Design review of the part shown in the three views and the two pictorial views. Dimensions are in mm from the part's minimum x, y and z. A direction names the side the tool comes from. Coordinates: 2 decimals unless noted, no trailing zeros. Write each loop counter-clockwise with the first axis right and the second up, starting at its lowest first coordinate (ties: lowest second). Pieces come first, ordered by that corner, then holes. Notation, with made-up numbers: (72, -33.5) -> (128, -33.5) arc R35 cw to (128, -0.5) -> close; hole circle Ø2 at (-34, 19). An arc over 180 degrees is marked (long way). Write item = value, one per line. Start each with the question number.
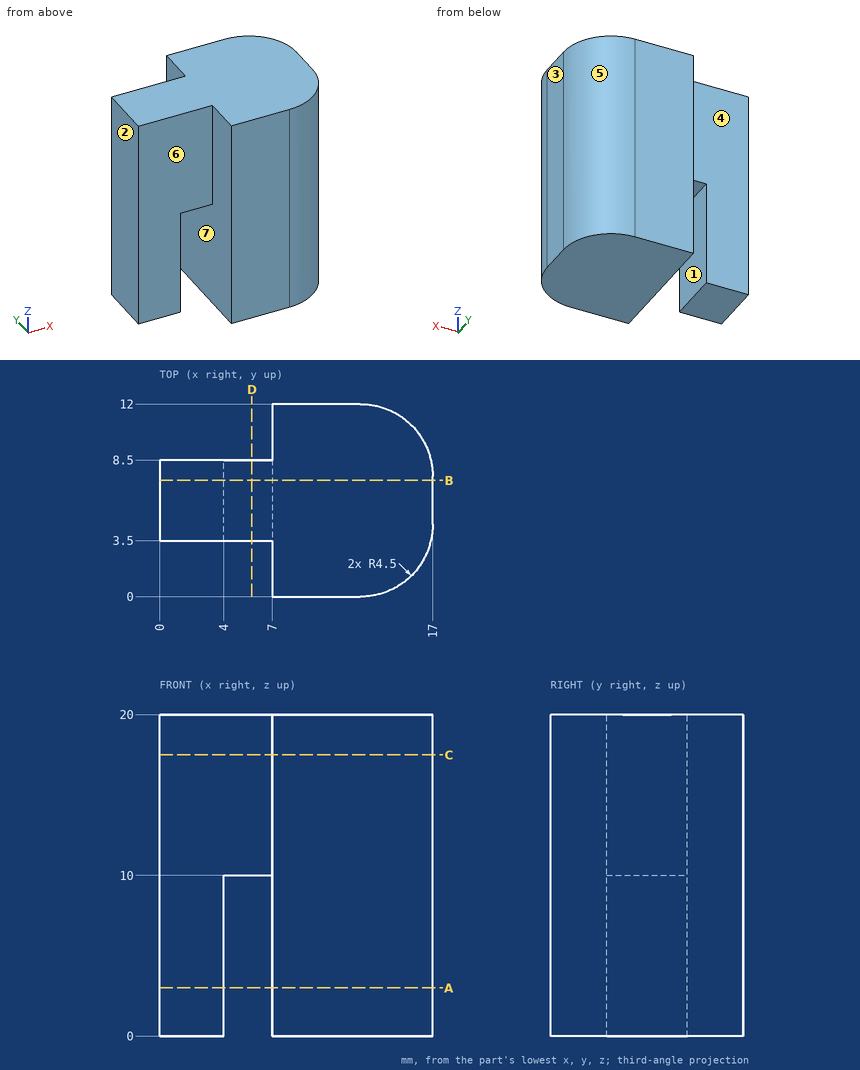
(1) Mouldability with a two-part tool opening along X and no side actions: class the marked faces 1, 2, 3 and 4 as pulls with the +X half, pulls with the -X half, needs draft (parallel to the pull), parting line crosses it, or undercut.
(2) Take a section at C-C, the plane z = 17.5. State the section outline as (x, y) points.
(3) For the marked faces 5, 6 and 7, list the 3-axis set-ups (+Z, -Z, +X, -X, +Y, -Y) from which the entire face can be reached by the end or side of a thin tool; tool diameter is ignored.
(4) For line 1 (X direction, y = 7, z = 3); line 2 (Y direction, x = 3.75, z = 2.25); line 3 (Y direction, x = 13.5, z = 14.5), list the stretches that pass through material, from the lowest coordinate up.
(5) For pin 1 Ø2 at (y, z) = (10.5, 8.5) entering from -X, flat-tipped, find the tip position at first contact; note if it passes through.
(6) Take a section at D-D, the plane x = 5.75. State the section outline as (y, z) points.
(7) Take a section at B-B, the plane y = 7.25. State the section outline as (x, z) points, then the cut area to 3 significant figures.
(8) Take a section at A-A, the plane z = 3. State the section outline as (x, y) points.
Report:
q1.face_1 = undercut
q1.face_2 = pulls with the -X half
q1.face_3 = pulls with the +X half
q1.face_4 = needs draft
q2.outline = (0, 3.5) -> (7, 3.5) -> (7, 0) -> (12.5, 0) arc R4.5 ccw to (17, 4.5) -> (17, 7.5) arc R4.5 ccw to (12.5, 12) -> (7, 12) -> (7, 8.5) -> (0, 8.5) -> close
q3.face_5 = +Z, -Z, +X, +Y
q3.face_6 = +Z, -Z, -X, -Y
q3.face_7 = -Z
q4.line_1 = 0 to 4, 7 to 17
q4.line_2 = 3.5 to 8.5
q4.line_3 = 0.11 to 11.89
q5.pin_1 = 7
q6.outline = (3.5, 10) -> (8.5, 10) -> (8.5, 20) -> (3.5, 20) -> close
q7.outline = (0, 0) -> (4, 0) -> (4, 10) -> (7, 10) -> (7, 0) -> (17, 0) -> (17, 20) -> (0, 20) -> close
q7.area = 310 mm2
q8.outline = (0, 3.5) -> (4, 3.5) -> (4, 8.5) -> (0, 8.5) -> close; (7, 0) -> (12.5, 0) arc R4.5 ccw to (17, 4.5) -> (17, 7.5) arc R4.5 ccw to (12.5, 12) -> (7, 12) -> close
